Geometry: final body of the model. Coordinates: model frame, mm. Face numbers are marked on the shaded views. Give positions to 0.01 mm unless a question says otherwise; leave off trailing zeros. Write each loop counter-clockwise with the first axis right and the second up, starting at its lowest first coordinate (ties: lowest second). Pieces come first, ordered by that corner, then holes.
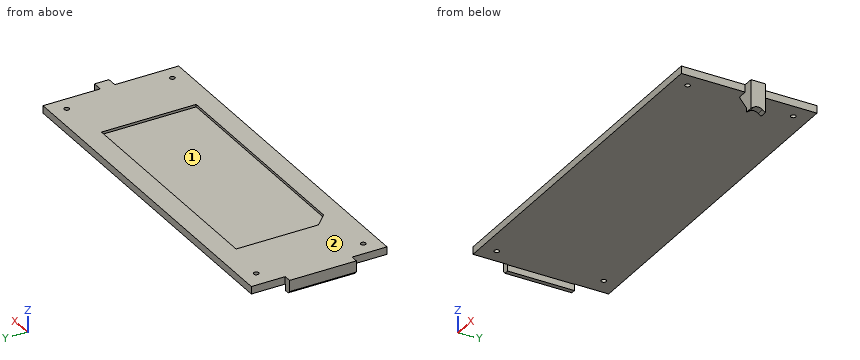
from build123d import *

# Parameters (mm, degrees)
F0_W      = 143.9
F0_H      = 54.4
F1_DEPTH  = 3
F2_W      = 5.8
F2_H      = 3
F3_DEPTH  = 4
F4_W      = 4
F4_H      = 5.8
F5_DEPTH  = 8.5
F7_DEPTH  = 5
F8_R      = 3
F9_W      = 26.8
F9_H      = 3
F10_DEPTH = 3
F11_W     = 3
F11_H     = 26.8
F12_DEPTH = 2.5
F13_W     = 26.8
F13_H     = 2.5
F14_DEPTH = 0.2
F16_DEPTH = 1
F17_W     = 5.8
F17_H     = 12.271342
F18_DEPTH = 1
F20_DEPTH = 5.8
F21_SIZE  = 1
F22_R     = 1
F23_DEPTH = 3


with BuildPart() as f1:
    # F0 (on Top) → F1 (new body)
    with BuildSketch(Plane.XY):
        with Locations((71.95, -27.2)):
            Rectangle(F0_W, F0_H)
    extrude(amount=F1_DEPTH)

    # F2 (on face) → F3 (join)
    with BuildSketch(Plane.YZ.offset(143.9)):
        with Locations((-25.9, 1.5)):
            Rectangle(F2_W, F2_H)
    extrude(amount=F3_DEPTH)

    # F4 (on face) → F5 (join)
    with BuildSketch(Plane(origin=(0, 0, 0), x_dir=(1, 0, 0), z_dir=(0, 0, -1))):
        with Locations((145.9, 25.9)):
            Rectangle(F4_W, F4_H)
    extrude(amount=F5_DEPTH)

    # F6 (on face) → F7 (cut)
    with BuildSketch(Plane.YZ.offset(147.9)):
        Polygon((-25.9, -6.469398), (-28.8, -8.5), (-23, -8.5), align=None)
    extrude(amount=-F7_DEPTH, mode=Mode.SUBTRACT)

    # F8
    f8_edges = [f1.edges().sort_by_distance(p)[0] for p in [
        (145.9, -25.9, -6.469398),
    ]]
    fillet(f8_edges, radius=F8_R)

    # F9 (on face) → F10 (join)
    with BuildSketch(Plane(origin=(0, 0, 0), x_dir=(0, -1, 0), z_dir=(-1, 0, 0))):
        with Locations((27, 1.5)):
            Rectangle(F9_W, F9_H)
    extrude(amount=F10_DEPTH)

    # F11 (on face) → F12 (join)
    with BuildSketch(Plane(origin=(0, 0, 0), x_dir=(1, 0, 0), z_dir=(0, 0, -1))):
        with Locations((-1.5, 27)):
            Rectangle(F11_W, F11_H)
    extrude(amount=F12_DEPTH)

    # F13 (on face) → F14 (cut)
    with BuildSketch(Plane.YZ):
        with Locations((-27, -1.25)):
            Rectangle(F13_W, F13_H)
    extrude(amount=-F14_DEPTH, mode=Mode.SUBTRACT)

    # F15 (on face) → F16 (cut)
    with BuildSketch(Plane.XY.offset(3)):
        Polygon((118, -8.4), (25, -8.4), (25, -41.4), (30, -46.4), (118, -46.4), align=None)
    extrude(amount=-F16_DEPTH, mode=Mode.SUBTRACT)

    # F17 (on face) → F18 (cut)
    with BuildSketch(Plane(origin=(143.9, 0, 0), x_dir=(0, -1, 0), z_dir=(-1, 0, 0))):
        with Locations((25.9, -6.135671)):
            Rectangle(F17_W, F17_H)
    extrude(amount=-F18_DEPTH, mode=Mode.SUBTRACT)

    # F19 (on face) → F20 (join)
    with BuildSketch(Plane(origin=(0, -23, 0), x_dir=(-1, 0, 0), z_dir=(0, 1, 0))):
        Polygon((-139.9, 0), (-144.9, 0), (-144.9, -7), align=None)
    extrude(amount=-F20_DEPTH)

    # F21
    f21_edges = [f1.edges().sort_by_distance(p)[0] for p in [
        (-3, -27, -2.5),
    ]]
    chamfer(f21_edges, length=F21_SIZE)

    # F22 (on face) → F23 (cut)
    with BuildSketch(Plane.XY.offset(3)):
        with Locations((137.9, -48.4)):
            Circle(F22_R)
        with Locations((137.9, -6)):
            Circle(F22_R)
        with Locations((6.019338, -48.4)):
            Circle(F22_R)
        with Locations((7, -6)):
            Circle(F22_R)
    extrude(amount=-F23_DEPTH, mode=Mode.SUBTRACT)


solid = f1.part
Q1. Section A-A on y = -39. Output: boundary loops of the cut face in (x, z), plus the area to 3 significant figures.
Filled sheet:
outline: (-3, -1.5) - (-2, -2.5) - (-0.2, -2.5) - (-0.2, 0) - (143.9, 0) - (143.9, 3) - (118, 3) - (118, 2) - (25, 2) - (25, 3) - (-3, 3) - close
area: 354 mm2
Q2. Pull-direction query (X, two-part tool) for the marked faces 1 and 2; classes: released by +X, released by -X, zero draft, split by the parting line, or undercut.
Filled sheet:
face 1: undercut
face 2: zero draft
Q3. Ray query, line 1 along Y through (x, z) = (137.9, 1.4); line 2 along Y through (x, z) = (6.5, 0.5); line 3 along Z through (x, y) = (98, -36). Return the intervals inside material, ascending.
Filled sheet:
line 1: y = -54.4 to -49.4, -47.4 to -7, -5 to 0
line 2: y = -54.4 to -49.28, -47.52 to -6.87, -5.13 to 0
line 3: z = 0 to 2
Q4. Pin query (flat end, axial travel): P1, Ø1.5, axis at y = -4, z = 1, coming from the -X side; P2, Ø2.5, axis at x = 144.5, z = -4, coming from the -Y side; P3, Ø10, axis at x = 103.5, y = -39, coming from the +Z side; P4, Ø1.6, axis at x = 6.02, y = -48.4, coming from the +Z side. Return the tip coordinate at first contact, or that it passes through.
Filled sheet:
P1: stops at x = 0
P2: stops at y = -28.8
P3: stops at z = 2
P4: passes through
Q5. Section B-B on x = 109.5. Output: boundary loops of the cut face in (y, z), plus the area to 3 significant figures.
Filled sheet:
outline: (-54.4, 0) - (0, 0) - (0, 3) - (-8.4, 3) - (-8.4, 2) - (-46.4, 2) - (-46.4, 3) - (-54.4, 3) - close
area: 125 mm2
Q6. Section C-C on z = -4.25. Output: boundary loops of the cut face in (x, y), plus the area to 3 significant figures.
Filled sheet:
outline: (142.94, -28.8) - (147.9, -28.8) - (147.9, -23) - (142.94, -23) - close
area: 28.8 mm2
